Autodesk Fusion 360 part; units mm, degrees
sketch "Sketch1" plane through (0, 0, 0) normal (0, 0, 1) x (1, 0, 0)
  circle A0 centre (0, 0) radius 87.5
  circle A1 centre (0, 0) radius 77.5
  line L0 (77.5, 0) -> (97.5, 0)
  line L1 (97.5, 0) -> (97.5, -97.5)
  line L2 (97.5, -97.5) -> (77.5, -97.5)
  line L3 (77.5, -97.5) -> (77.5, 0)
  line L4 (-77.5, 0) -> (-97.5, 0)
  line L5 (-97.5, 0) -> (-97.5, -97.5)
  line L6 (-97.5, -97.5) -> (-77.5, -97.5)
  line L7 (-77.5, -97.5) -> (-77.5, 0)
  line L8 (97.5, -97.5) -> (-97.5, -97.5)
  line L9 (-97.5, -97.5) -> (-97.5, -102.5)
  line L10 (-97.5, -102.5) -> (97.5, -102.5)
  line L11 (97.5, -102.5) -> (97.5, -97.5)
  dimension "d1" = 155
  dimension "d2" = 175
  dimension "d15" = 97.5
  dimension "d16" = 5
  dimension "d17" = 10
  dimension "d18" = 20
  dimension "d19" = 20
extrude "Extrude1" add sketch "Sketch1" along normal blind 15 contours A0 L0 L1 L2 L3 L8 | A0 L0 L3 | A0 L4 L7 | A0 L4 L5 L6 L7 L8 | A0 L3 L7 L8 | A0 A1 L3 L7 | L2 L6 L8 L9 L10 L11
sketch "Sketch2" plane through (0, 0, 0) normal (0, 0, 1) x (1, 0, 0)
  circle A0 centre (0, 0) radius 80.5
  dimension "d10" = 161
extrude "Extrude2" cut sketch "Sketch2" along normal blind 5.5 from surface at 4
sketch "Sketch3" plane through (0, 0, 15) normal (0, 0, 1) x (-1, 0, 0)
  line L0 (77.5, 0) -> (97.5, 0)
  line L1 (97.5, 0) -> (97.5, 102.5)
  line L2 (97.5, 102.5) -> (-97.5, 102.5)
  line L3 (-97.5, 102.5) -> (-97.5, 0)
  line L4 (-97.5, 0) -> (-77.5, 0)
  arc A0 (77.5, 0) -> (-77.5, 0) centre (0, 0) ccw
  line L5 (-30, 102.5) -> (30, 102.5)
  line L6 (30, 102.5) -> (30, 97.5)
  line L7 (30, 97.5) -> (-30, 97.5)
  line L8 (-30, 97.5) -> (-30, 102.5)
  dimension "d22" = 30
  dimension "d23" = 30
extrude "Extrude3" add sketch "Sketch3" along normal blind 30 contours L2 L5 L6 L7 L8
fillet "Fillet2" radius 15 4 edges at (-30, -100, 45) (30, -100, 45) (-30, -100, 15) (30, -100, 15)
sketch "Sketch4" plane through (0, -97.5, 0) normal (0, 1, 0) x (-1, 0, 0)
  arc A0 (-15, 45) -> (-30, 30) centre (-15, 30) ccw
  arc A1 (-45, 15) -> (-30, 30) centre (-45, 30) ccw
  line L0 (-45, 15) -> (45, 15)
  arc A2 (30, 30) -> (45, 15) centre (45, 30) ccw
  arc A3 (30, 30) -> (15, 45) centre (15, 30) ccw
  line L1 (15, 45) -> (-15, 45)
  line L2 (-97.5, 7.5) -> (97.5, 7.5) construction
  line L3 (-45, 0) -> (45, 0)
  line L4 (15, -30) -> (-15, -30)
  arc A4 (15, -30) -> (30, -15) centre (15, -15) ccw
  arc A5 (45, 0) -> (30, -15) centre (45, -15) ccw
  arc A6 (-30, -15) -> (-15, -30) centre (-15, -15) ccw
  arc A7 (-30, -15) -> (-45, 0) centre (-45, -15) ccw
  point P0 (0, 30)
  point P1 (-97.5, 7.5)
  point P2 (97.5, 7.5)
  point P3 (0, -15)
  dimension "d28" = 15
sketch "Sketch5" plane through (0, 0, 0) normal (0, 0, -1) x (1, 0, 0)
  line L0 (-97.5, 0) -> (-77.5, 0)
  arc A0 (77.5, 0) -> (-77.5, 0) centre (0, 0) ccw
  line L1 (77.5, 0) -> (97.5, 0)
  line L2 (97.5, 0) -> (97.5, 102.5)
  line L3 (97.5, 102.5) -> (-97.5, 102.5)
  line L4 (-97.5, 102.5) -> (-97.5, 0)
  line L5 (80, 102.5) -> (-80, 102.5)
  line L6 (-80, 102.5) -> (-80, 97.5)
  line L7 (-80, 97.5) -> (80, 97.5)
  line L8 (80, 97.5) -> (80, 102.5)
  dimension "d39" = 80
  dimension "d40" = 80
extrude "Extrude4" add sketch "Sketch5" along normal blind 30 contours L3 L5 L6 L7 L8
fillet "Fillet4" radius 15 4 edges at (80, -100, -30) (-80, -100, -30) (-80, -100, 0) (80, -100, 0)
sketch "Sketch6" plane through (0, -97.5, 0) normal (0, 1, 0) x (-1, 0, 0)
  arc A0 (65, -30) -> (80, -15) centre (65, -15) ccw
  arc A1 (95, 0) -> (80, -15) centre (95, -15) ccw
  line L0 (95, 0) -> (-95, 0)
  arc A2 (-80, -15) -> (-95, 0) centre (-95, -15) ccw
  arc A3 (-80, -15) -> (-65, -30) centre (-65, -15) ccw
  line L1 (-65, -30) -> (65, -30)
  line L2 (-77.5, 15) -> (77.5, 15)
  point P0 (0, -20)
  point P1 (0, 35)
  point P2 (50, -20)
  point P3 (-50, -20)
  dimension "d49" = 20
  dimension "d50" = 20
  dimension "d53" = 50
  dimension "d54" = 50
hole "Hole2" at (0, -97.5, -20) at (0, -97.5, 35) at (-50, -97.5, -20) at (50, -97.5, -20) direction (0, -1, 0) diameter 4 end through all countersink diameter 4.4 countersink angle 90
sketch "Sketch7" plane through (0, 0, 0) normal (0, 1, 0) x (-1, 0, 0)
  line L0 (77.5, 9.5) -> (80.5, 9.5)
  line L1 (80.5, 9.5) -> (80.5, 4)
  line L2 (80.5, 4) -> (77.5, 4)
  line L3 (77.5, 4) -> (77.5, 0)
  line L4 (77.5, 0) -> (97.5, 0)
  line L5 (97.5, 0) -> (97.5, 15)
  line L6 (97.5, 15) -> (77.5, 15)
  line L7 (77.5, 15) -> (77.5, 9.5)
  line L8 (-77.5, 0) -> (-97.5, 0)
  line L9 (-97.5, 0) -> (-97.5, 15)
  point P0 (90, 7.5)
  point P1 (-90, 7.5)
  dimension "d55" = 7.5
  dimension "d56" = 7.5
  dimension "d57" = 7.5
  dimension "d58" = 7.5
hole "Hole3" at (-90, 0, 7.5) at (90, 0, 7.5) direction (0, -1, 0) diameter 3.5 depth 50 tip angle 180
fillet "Fillet5" radius 10 2 edges at (0, -97.5, 0) (0, -97.5, 15)
equation "d15 = d2 / 2 + 10 mm"
equation "d18 = d17 + 10 mm"
equation "d19 = d18"
equation "d23 = d22"
equation "d40 = d39"
equation "d56 = d55"
equation "d58 = d57"
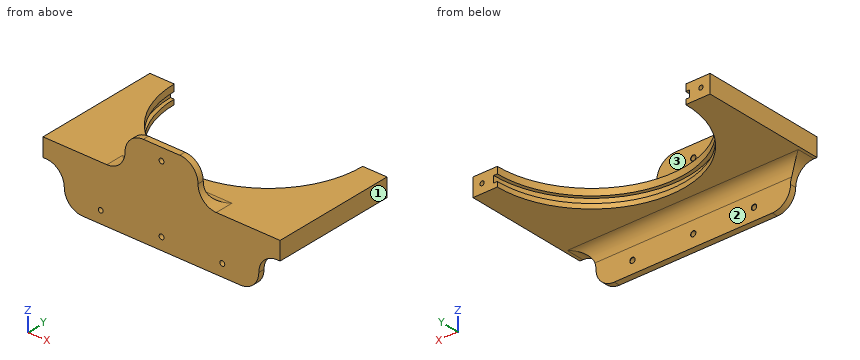
Work out the finished part from the listing and answer in its coordinate system (mm). Face numbers are marked on the shaded views. A direction names the side the tool comes from. Give positions to 0.01 mm unless a question says otherwise; leave off trailing zeros. Order: outer loops, then holes, each group sorted by start corner. A loop starts at its lowest first (then second) coordinate and runs counter-clockwise, first axis right, second up.
1. Straight lines are drawn through the part: L1, parallel to Z at x = 0, y = -99; L2, parallel to Z at x = -50, y = -101.05; L3, parallel to X at y = -100.75, z = -20. For each, find the intervals that lie inside material, in ascending order.
Result sheet:
L1: z = -30 to -22, -18 to 33, 37 to 45
L2: z = -30 to -22, -18 to 15
L3: x = -79.14 to -52, -48 to -2, 2 to 48, 52 to 79.14
2. Section B-B, the plane y = -9 is taken. Determine the outline of the cut face in (x, z).
Result sheet:
outline: (-97.5, 0) - (-76.98, 0) - (-76.98, 4) - (-80, 4) - (-80, 9.5) - (-76.98, 9.5) - (-76.98, 15) - (-97.5, 15) - close; (76.98, 0) - (97.5, 0) - (97.5, 15) - (76.98, 15) - (76.98, 9.5) - (80, 9.5) - (80, 4) - (76.98, 4) - close; hole circle Ø3.5 at (-90, 7.5); hole circle Ø3.5 at (90, 7.5)
3. Each of these flat-tipped pins is pushed along its axis until it touches: P1, Ø6, axis at x = 7, z = 38, coming from the +Y side; P2, Ø3, axis at x = 0, z = -20, coming from the -Y side; P3, Ø2, axis at x = -47.5, z = -3.5, coming from the +Y side. Where does it stop, or does it pass through?
Result sheet:
P1: stops at y = -97.5
P2: passes through
P3: stops at y = -94.11
4. Section C-C, the plane z = -20 is taken. Determine the outline of the cut face in (x, y), and give its area (3 significant figures).
Result sheet:
outline: (-79.14, -102.5) - (-52, -102.5) - (-52, -97.7) - (-52.2, -97.5) - (-79.14, -97.5) - close; (-48, -102.5) - (-2, -102.5) - (-2, -97.7) - (-2.2, -97.5) - (-47.8, -97.5) - (-48, -97.7) - close; (2, -102.5) - (48, -102.5) - (48, -97.7) - (47.8, -97.5) - (2.2, -97.5) - (2, -97.7) - close; (52, -102.5) - (79.14, -102.5) - (79.14, -97.5) - (52.2, -97.5) - (52, -97.7) - close
area: 731 mm2
5. For the marked faces 1, 2 and 3, determine the directions among +Z, -Z, +X, -X, +Y, -Y from which every point of the face is accessible in a straight line to the end or side of a thin tool.
Result sheet:
face 1: +Z, -Z, +X, +Y, -Y
face 2: -Z, +X, -X, +Y
face 3: +Z, +X, -X, +Y
6. Section D-D, the plane z = 11.5 is taken. Determine the outline of the cut face in (x, y), and give its area (3 significant figures).
Result sheet:
outline: (-97.5, -102.5) - (97.5, -102.5) - (97.5, 0) - (77.5, 0) arc R77.5 cw to (-77.5, 0) - (-97.5, 0) - close
area: 10,600 mm2
7. Section A-A, the plane x = 0 is taken. Determine the outline of the cut face in (y, z), and give its area (3 significant figures).
Result sheet:
outline: (-102.5, -30) - (-97.5, -30) - (-97.5, -22.2) - (-97.7, -22) - (-102.5, -22) - close; (-102.5, -18) - (-97.7, -18) - (-97.5, -17.8) - (-97.5, -10) arc R10 cw to (-87.5, 0) - (-77.5, 0) - (-77.5, 4) - (-80.5, 4) - (-80.5, 9.5) - (-77.5, 9.5) - (-77.5, 15) - (-87.5, 15) arc R10 cw to (-97.5, 25) - (-97.5, 32.8) - (-97.7, 33) - (-102.5, 33) - close; (-102.5, 37) - (-97.7, 37) - (-97.5, 37.2) - (-97.5, 45) - (-102.5, 45) - close
area: 661 mm2
